Verification items for this drawing (mm, ordinates from the low corner). Coordinates: 2 decimals unless noted, no trailing zeros. Loops run counter-clockwise (first coordinate to the right, second up) from the corner with the lowest first, then second, coordinate; pieces in that order, holes last.
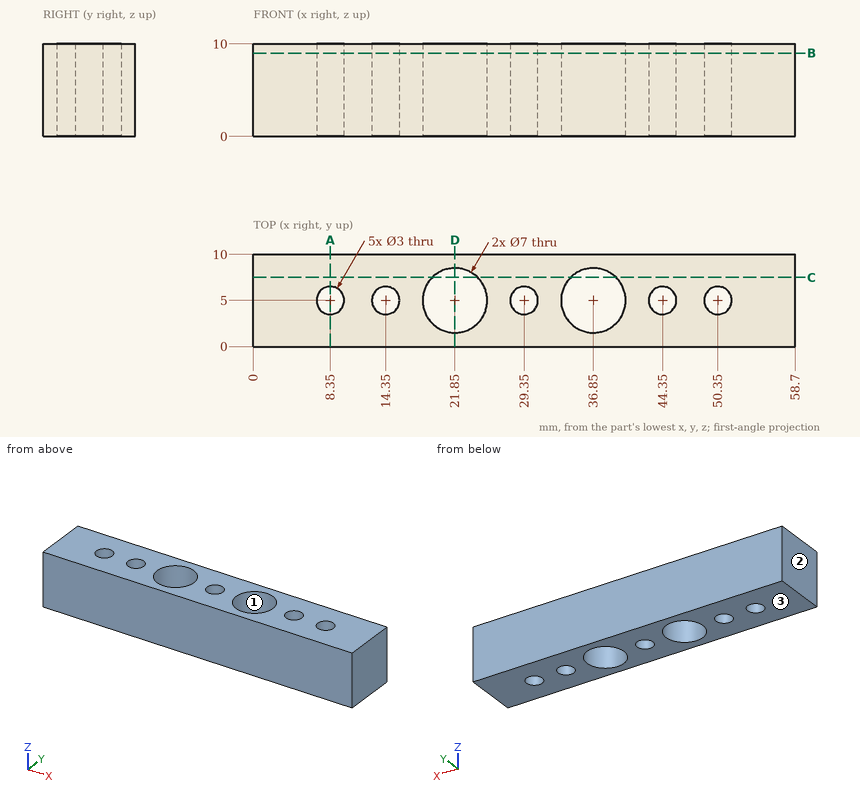
(1) Section check C-C, the plane y = 7.5. Enter the section's corners in (x, z).
(2) Section check D-D, the plane x = 21.85. Enter the section's corners in (y, z), plus the area to 3 significant figures.
(3) Section check B-B, the plane z = 9. Enter the section's corners in (x, y).
(4) Section check A-A, the plane x = 8.35. Enter the section's corners in (y, z), plus the area to 3 significant figures.
(5) Scan lines: line 1 along Y through (x, z) = (36.85, 3); line 2 along Y through (x, z) = (50.35, 7.5); line 3 along X through (y, z) = (8, 5.25). Record each from-to range of solid material in increasing order.
(6) Draft check along X on the marked faces 1, 2 and 3. Enter one of: pulls with the +X half, pulls with the -X half, needs draft (parallel to the pull), parting line crosses it, or undercut.
Determined:
1. outline: (0, 0) - (19.4, 0) - (19.4, 10) - (0, 10) - close; (24.3, 0) - (34.4, 0) - (34.4, 10) - (24.3, 10) - close; (39.3, 0) - (58.7, 0) - (58.7, 10) - (39.3, 10) - close
2. outline: (0, 0) - (1.5, 0) - (1.5, 10) - (0, 10) - close; (8.5, 0) - (10, 0) - (10, 10) - (8.5, 10) - close
2. area: 30.0 mm2
3. outline: (0, 0) - (58.7, 0) - (58.7, 10) - (0, 10) - close; hole circle Ø3 at (8.35, 5); hole circle Ø3 at (14.35, 5); hole circle Ø7 at (21.85, 5); hole circle Ø3 at (29.35, 5); hole circle Ø7 at (36.85, 5); hole circle Ø3 at (44.35, 5); hole circle Ø3 at (50.35, 5)
4. outline: (0, 0) - (3.5, 0) - (3.5, 10) - (0, 10) - close; (6.5, 0) - (10, 0) - (10, 10) - (6.5, 10) - close
4. area: 70.0 mm2
5. line 1: y = 0 to 1.5, 8.5 to 10
5. line 2: y = 0 to 3.5, 6.5 to 10
5. line 3: x = 0 to 20.05, 23.65 to 35.05, 38.65 to 58.7
6. face 1: undercut
6. face 2: pulls with the -X half
6. face 3: needs draft
